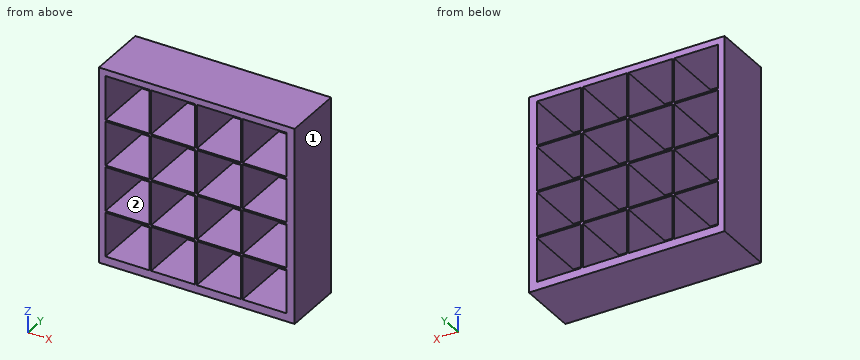
from build123d import *

# Parameters (mm, degrees)
F0_W     = 1200
F0_H     = 370
F1_DEPTH = 1200
F2_W     = 270
F2_H     = 270
F3_DEPTH = 370.001


with BuildPart() as f1:
    # F0 (on Top) → F1 (new body)
    with BuildSketch(Plane.XY):
        with Locations((536.95002, 123.801892)):
            Rectangle(F0_W, F0_H)
    extrude(amount=F1_DEPTH)

    # F2 (on face) → F3 (cut, through all)
    with BuildSketch(Plane.XZ.offset(61.198108)):
        with Locations((111.95002, 1025)):
            Rectangle(F2_W, F2_H)
        with Locations((391.95002, 1025)):
            Rectangle(F2_W, F2_H)
        with Locations((671.95002, 1025)):
            Rectangle(F2_W, F2_H)
        with Locations((951.95002, 1025)):
            Rectangle(F2_W, F2_H)
        with Locations((951.95002, 745)):
            Rectangle(F2_W, F2_H)
        with Locations((671.95002, 745)):
            Rectangle(F2_W, F2_H)
        with Locations((391.95002, 745)):
            Rectangle(F2_W, F2_H)
        with Locations((111.95002, 745)):
            Rectangle(F2_W, F2_H)
        with Locations((111.95002, 465)):
            Rectangle(F2_W, F2_H)
        with Locations((391.95002, 465)):
            Rectangle(F2_W, F2_H)
        with Locations((671.95002, 465)):
            Rectangle(F2_W, F2_H)
        with Locations((951.95002, 465)):
            Rectangle(F2_W, F2_H)
        with Locations((951.95002, 185)):
            Rectangle(F2_W, F2_H)
        with Locations((671.95002, 185)):
            Rectangle(F2_W, F2_H)
        with Locations((391.95002, 185)):
            Rectangle(F2_W, F2_H)
        with Locations((111.95002, 185)):
            Rectangle(F2_W, F2_H)
    extrude(amount=-F3_DEPTH, mode=Mode.SUBTRACT)


solid = f1.part
Read the model definition and answer for the solid it produces. Units are mm, in the model's axes. Face numbers are marked on the shaded views. Give positions to 0.01 mm unless a question says otherwise; leave off trailing zeros. Loops run counter-clockwise (first coordinate to the right, second up) from the corner with the lowest first, then second, coordinate; pieces in that order, holes last. Notation, with made-up numbers: M -32.75,65.5 L 14.25,65.5 A19 cw 14.25,76.5 Z; hole C -27.75,2 d9. An arc over 180 degrees is marked long. Write each question's results on one line, items separated by ' | '.
1. Section C-C on y = -32 is taken. State how many separate pieces and enclosed holes the cut face has, plus the area to 3 significant figures.
Values:
separate pieces: 1 | enclosed holes: 16 | area: 274,000 mm^2
2. Section A-A on x = 937 is taken. Give the vertices of the cut face in (y, z).
Values:
outline: M -61.2,0 L 308.8,0 L 308.8,50 L -61.2,50 Z; M -61.2,320 L 308.8,320 L 308.8,330 L -61.2,330 Z; M -61.2,600 L 308.8,600 L 308.8,610 L -61.2,610 Z; M -61.2,880 L 308.8,880 L 308.8,890 L -61.2,890 Z; M -61.2,1160 L 308.8,1160 L 308.8,1200 L -61.2,1200 Z
3. The mould has two halves that part along X. Classify the marked faces 1 and 2: pulls with the +X half, pulls with the -X half, needs draft (parallel to the pull), parting line crosses it, or undercut.
Values:
face 1: pulls with the +X half | face 2: undercut
4. Straight lines are drawn through the part: line 1 (Z direction, x = 611.5, y = 237); line 2 (X direction, y = -35, z = 226). For each, find the intervals that lie inside material, in ascending order. Write a range as [from, to].
Values:
line 1: z = [0, 50], [320, 330], [600, 610], [880, 890], [1160, 1200] | line 2: x = [-63.05, -23.05], [246.95, 256.95], [526.95, 536.95], [806.95, 816.95], [1086.95, 1136.95]
5. Section B-B on z = 1016 is taken. Give the vertices of the cut face in (x, y).
Values:
outline: M -63.05,-61.2 L -23.05,-61.2 L -23.05,308.8 L -63.05,308.8 Z; M 246.95,-61.2 L 256.95,-61.2 L 256.95,308.8 L 246.95,308.8 Z; M 526.95,-61.2 L 536.95,-61.2 L 536.95,308.8 L 526.95,308.8 Z; M 806.95,-61.2 L 816.95,-61.2 L 816.95,308.8 L 806.95,308.8 Z; M 1086.95,-61.2 L 1136.95,-61.2 L 1136.95,308.8 L 1086.95,308.8 Z
